Build history of the part. All positions in model axes, mm. Face numbers are marked on the shaded views. A direction names the side the tool comes from. Round coordinates to 2 decimals unless told otherwise and drop trailing zeros. Loops run counter-clockwise (first coordinate to the right, second up) from the corner with the lowest first, then second, coordinate; pieces in that order, holes last.
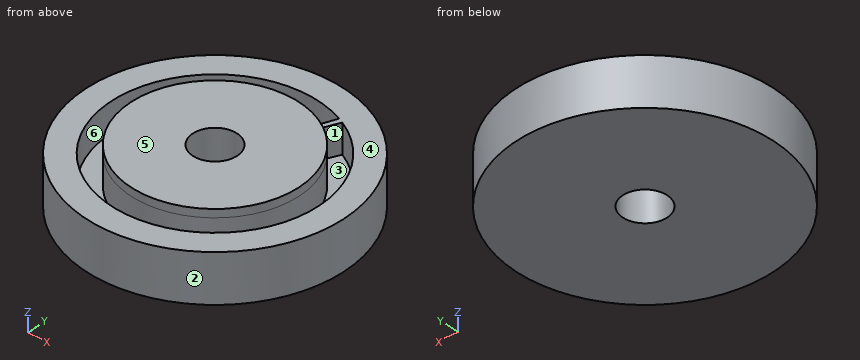
from build123d import *

# Parameters (mm, degrees)
SKETCH1_R           = 23.75
BOSS_EXTRUDE1_DEPTH = 8.9
SKETCH3_R           = 15.5
BOSS_EXTRUDE2_DEPTH = 10.4
CUT_EXTRUDE1_START  = 5.4
CUT_EXTRUDE1_DEPTH  = 5.4
CUT_EXTRUDE2_REACH  = 37.161
SKETCH5_R           = 4.08


with BuildPart() as part:
    # Sketch1 → Boss-Extrude1 (new body)
    with BuildSketch(Plane.XY):
        Circle(SKETCH1_R)
    extrude(amount=BOSS_EXTRUDE1_DEPTH)

    # Sketch3 → Boss-Extrude2 (add)
    with BuildSketch(Plane(origin=(0, 0, 0), x_dir=(-1, 0, 0), z_dir=(0, 0, -1))):
        Circle(SKETCH3_R)
    extrude(amount=-BOSS_EXTRUDE2_DEPTH)

    # Sketch4 → Cut-Extrude1 (cut)
    with BuildSketch(Plane(origin=(0, 0, 8.9), x_dir=(-1, 0, 0), z_dir=(0, 0, -1)).offset(CUT_EXTRUDE1_START)):
        with BuildLine():
            Line((-5.848746097, 14.354169049), (-7.167594485, 17.704112214))
            ThreePointArc((-7.167594485, 17.704112214), (7.650920777, -17.50066888), (-8.128479811, 17.284033556))
            Line((-8.128479811, 17.284033556), (-6.648360671, 14.001760617))
            ThreePointArc((-6.648360671, 14.001760617), (6.251037299, -14.183600836), (-5.848746097, 14.354169049))
        make_face()
    extrude(amount=-CUT_EXTRUDE1_DEPTH, mode=Mode.SUBTRACT)

    # Sketch5 → Cut-Extrude2 (cut, up to next)
    with BuildSketch(Plane.XY.offset(10.4), mode=Mode.PRIVATE) as cut_extrude2_sk1:
        Circle(SKETCH5_R)
    cut_extrude2_tool1 = extrude(cut_extrude2_sk1.sketch, amount=-CUT_EXTRUDE2_REACH, mode=Mode.PRIVATE) & part.part
    add(cut_extrude2_tool1.solids().sort_by_distance((0, 0, 10.4))[0], mode=Mode.SUBTRACT)


solid = part.part
(1) Pull direction X, two halves, no side cores. Call the marked faces 1, 2, 3 and 4: +X half, -X half, draft (parallel to the pull), parting line (faces both ways), or undercut.
Responses:
face 1: undercut
face 2: parting line
face 3: undercut
face 4: draft
(2) Slice it at C-C on z = 4.75. List the corners of the cut face in (x, y), plus the area to 3 significant figures.
Responses:
outline: circle Ø47.5 at (0, 0); hole circle Ø8.16 at (0, 0); hole (5.85, 14.35) - (7.17, 17.7) arc R19.1 ccw (long way) to (8.13, 17.28) - (6.65, 14) arc R15.5 cw (long way) to start
area: 1,330 mm2
(3) Probe line 1 (Y direction, x = 0, z = 8.25); line 2 (Y direction, x = 0, z = 3.25); line 3 (Y direction, x = 4.5, z = 6). List the from-to ranges inside material, lowest first.
Responses:
line 1: y = -23.75 to -19.1, -15.5 to -4.08, 4.08 to 15.5, 19.1 to 23.75
line 2: y = -23.75 to -4.08, 4.08 to 23.75
line 3: y = -23.32 to -18.56, -14.83 to 14.83, 18.56 to 23.32
(4) Slice it at D-D on z = 1.75. List the corners of the cut face in (x, y).
Responses:
outline: circle Ø47.5 at (0, 0); hole circle Ø8.16 at (0, 0)
(5) Pin check, flat tips, straight feed: P1, Ø6, axis at x = 18.5, z = 9, coming from the +Y side; P2, Ø6.5, axis at x = 0, y = 0, coming from the +Z side; P3, Ø5, axis at x = 11.5, z = 7.5, coming from the -Y side; P4, Ø2, axis at y = -4, z = 1.5, coming from the -X side. Stop position of each tip, or through.
Responses:
P1: stops at y = 17.99
P2: passes through
P3: stops at y = -21.98
P4: stops at x = -23.56
(6) Slice it at A-A on x = 0. List the corners of the cut face in (y, z).
Responses:
outline: (-23.75, 0) - (-4.08, 0) - (-4.08, 10.4) - (-15.5, 10.4) - (-15.5, 3.5) - (-19.1, 3.5) - (-19.1, 8.9) - (-23.75, 8.9) - close; (4.08, 0) - (23.75, 0) - (23.75, 8.9) - (19.1, 8.9) - (19.1, 3.5) - (15.5, 3.5) - (15.5, 10.4) - (4.08, 10.4) - close
(7) Which spindle directions (+Z, -Z, +X, -X, +Y, -Y) get a long thin tool onto all of the face, cutting with end or side? Do the marked faces 5 and 6. Say none if no direction does.
Responses:
face 5: +Z, +X, -X, +Y, -Y
face 6: +Z
